Autodesk Inventor part; units mm, degrees
ref_plane "YZ Plane" through (0, 0, 0) normal (1, 0, 0) x (0, 1, 0)
ref_plane "XZ Plane" through (0, 0, 0) normal (0, 1, 0) x (-1, 0, 0)
ref_plane "XY Plane" through (0, 0, 0) normal (0, 0, 1) x (1, 0, 0)
sketch "Sketch1" plane through (0, 0, 0) normal (0, 0, 1) x (1, 0, 0)
  circle A0 centre (0, 0) radius 2.5
  line L0 (-1.5, 2) -> (1.5, 2)
  circle A1 centre (0, 0) radius 5
  circle A2 centre (0, 0) radius 10
  dimension "d0" = 5
  dimension "d1" = 2
  dimension "d2" = 10
  dimension "d16" = 20
extrude "Extrusion1" add sketch "Sketch1" along normal blind 15 contours L0 A0 | A1 picked at (-0.3466, 2.0912)
extrude "Extrusion2" add sketch "Sketch1" against normal blind 3 contours L0 A0 | A1 | A2 picked at (-0.3466, 2.0912)
ref_plane "Work Plane2" through (0, 0, 0) normal (0, -1, 0) x (1, 0, 0)
ref_plane "Work Plane1" through (0, 5, 0) normal (0, -1, 0) x (1, 0, 0)
sketch "Sketch4" plane through (0, 0, 0) normal (0, -1, 0) x (1, 0, 0)
  line L0 (5, 15) -> (-5, 15)
  line L1 (-5, 15) -> (-10, 15)
  line L2 (-10, 15) -> (-10, 13.5)
  line L3 (-5, 0) -> (-5, 15)
  line L4 (-10, 13.5) -> (-5, 10.1834)
  line L5 (0, -6.6) -> (0, 18.6)
  point P0 (0, 0)
  dimension "d10" = 5
  dimension "d11" = 1.5
  dimension "d14" = 6
revolve "Revolution1" add sketch "Sketch4" angle 360 about axis through (0, 0, -10) along (0, 0, 1)
sketch "Sketch6" plane through (0, 0, -3) normal (0, 0, -1) x (-1, 0, 0)
  circle A0 centre (0, 0) radius 10
  circle A1 centre (-4.7517, -6.9277) radius 0.5
  line L0 (-5.0949, -6.5641) -> (-6.3365, -7.7362)
  line L1 (-4.4085, -7.2913) -> (-5.5187, -8.3393)
  dimension "d19" = 1
extrude "Extrusion3" cut sketch "Sketch6" against normal blind 3 contours L0 A1 L1 A0 | A1 picked at (-5.8735, -7.6008)
properties part number "D_coupler"
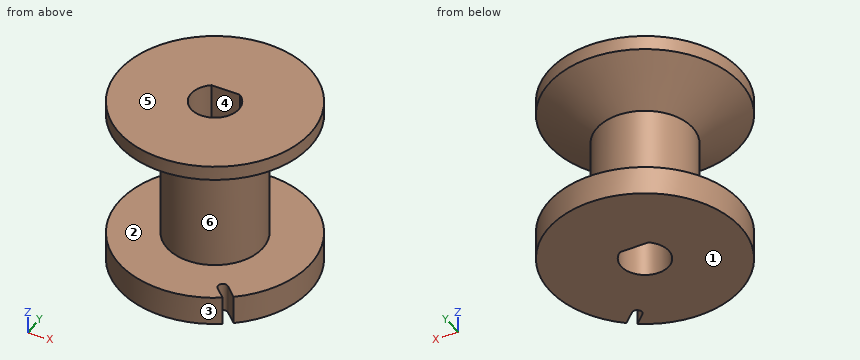
Work out the finished part from the listing and answer in its coordinate system (mm). Face numbers are marked on the shaded views. A direction names the side the tool comes from. Round coordinates to 2 decimals unless told otherwise and drop trailing zeros. Loops run counter-clockwise (first coordinate to the right, second up) from the corner with the lowest first, then second, coordinate; pieces in that order, holes last. Notation, with made-up numbers: M 16,83 L 65,83 A6 ccw 65,91 Z; hole C 20,-31 d7. An arc over 180 degrees is marked long. One line per question, with ' | ' between items. Start each with the question number.
(1) For a pull along Z with two mould halves and no side action, classify the marked faces 1, 2 and 3 as released by +Z, released by -Z, zero draft, split by the parting line, or undercut.
(2) A cutting plane is placed at A-A on y = 0. Write down the section's boundary in (x, z), plus the area to 3 significant figures.
(3) A cutting plane is placed at D-D on z = 12. Write down the section's boundary in (x, y).
(4) A cutting plane is placed at B-B on x = 0. Write down the section's boundary in (y, z).
(5) Flat-ended cylindrical pins translate along their axes: pin 1 Ø2 at (x, z) = (5, 4.5) entering from -Y; pin 2 Ø10 at (x, z) = (-7, 9) entering from +Y; pin 3 Ø1.5 at (x, z) = (-6.5, 6) entering from -Y; pin 4 Ø1.5 at (x, z) = (-3.5, 5) entering from +Y. Find the tip coordinate at first contact, or state that the pin passes through.
(6) A cutting plane is placed at C-C on z = -1.25. Write down the section's boundary in (x, y), plus the area to 3 significant figures.
(7) A tool of negligible diameter and unlimited length cuts with its end or side. For the marked faces 4, 5 and 6, from which of +Z, -Z, +X, -X, +Y, -Y can it reach the whole face along a straight path? Write none if from no direction.
(8) Find the intervals of material crossed by line 1 (Y direction, x = 0, z = 4.5); line 2 (X direction, y = 0, z = 1.5); line 3 (Y direction, x = -2.25, z = 14.25), in increasing order.
Geometry check:
1) face 1: released by -Z | face 2: undercut | face 3: zero draft
2) outline: M -10,-3 L -2.5,-3 L -2.5,15 L -10,15 L -10,13.5 L -5,10.18 L -5,0 L -10,0 Z; M 2.5,-3 L 10,-3 L 10,0 L 5,0 L 5,10.18 L 10,13.5 L 10,15 L 2.5,15 Z | area: 152 mm²
3) outline: C 0,0 d15.48; hole M -1.5,2 A2.5 ccw long 1.5,2 Z
4) outline: M -10,-3 L -2.5,-3 L -2.5,15 L -10,15 L -10,13.5 L -5,10.18 L -5,0 L -10,0 Z; M 2,-3 L 10,-3 L 10,0 L 5,0 L 5,10.18 L 10,13.5 L 10,15 L 2,15 Z
5) pin 1: stops at y = -3 | pin 2: stops at y = 8.76 | pin 3: passes through | pin 4: stops at y = 4.18
6) outline: M 4.41,-7.29 A0.5 cw 5.09,-6.56 L 6.34,-7.74 A10 ccw long 5.52,-8.34 Z; hole M -1.5,2 A2.5 ccw long 1.5,2 Z | area: 294 mm²
7) face 4: +Z, -Z | face 5: +Z, +X, -X, +Y, -Y | face 6: none
8) line 1: y = -5 to -2.5, 2 to 5 | line 2: x = -5 to -2.5, 2.5 to 5 | line 3: y = -9.74 to -1.09, 1.09 to 9.74
